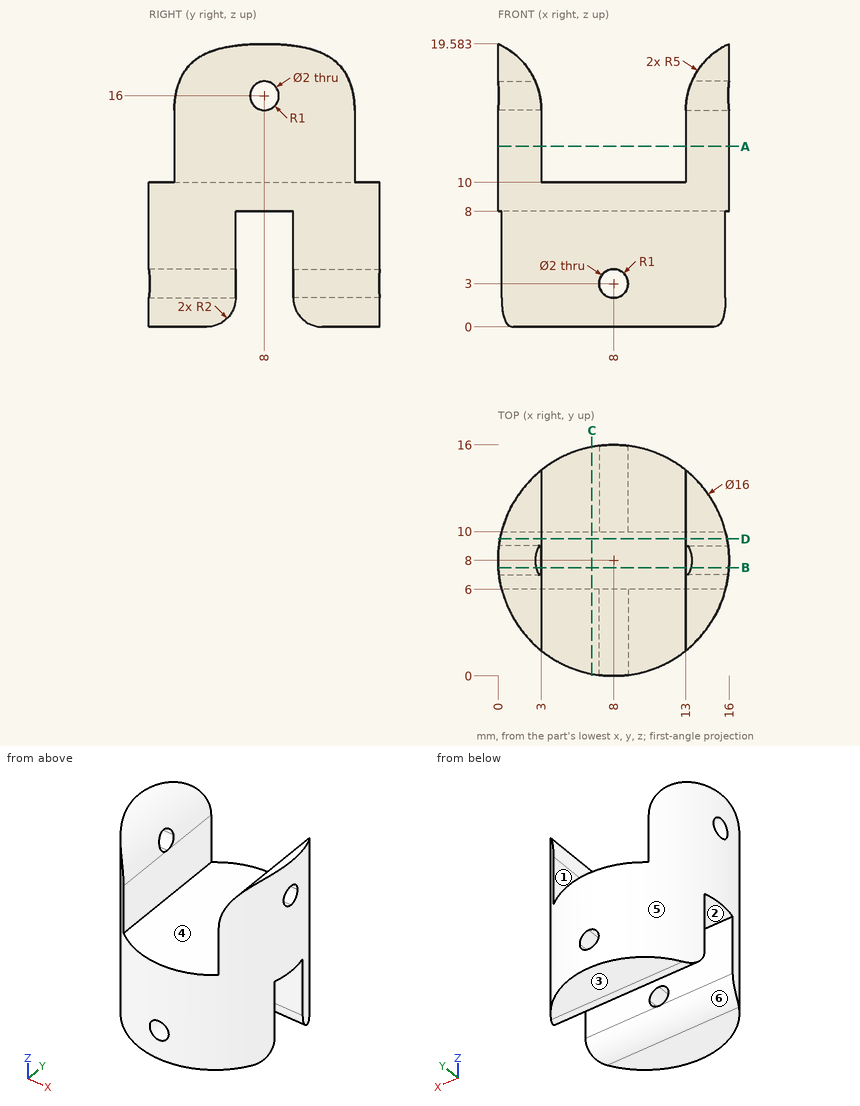
Study the drawing (mm; zero at the part's minimum x, y, z) and answer. A direction names the side the tool comes from. Coordinates: 2 decimals unless noted, no trailing zeros. Write each loop counter-clockwise with the first axis right and the second up, starting at its lowest first coordinate (ties: lowest second). Pieces come first, ordered by that corner, then holes. Notation, with made-up numbers: (23.5, 13) -> (47.5, 13) arc R4 cw to (47.5, 18) -> close; hole circle Ø4 at (3.25, 22.25). An arc over 180 degrees is marked (long way). Write item = value, one per line.
(1) Which of the six approach directions +Z, -Z, +X, -X, +Y, -Y give full straight-line access (tool end or side, diameter ignored) to the marked faces 1, 2 and 3?
From the geometry:
face_1 = +Z, +Y, -Y
face_2 = -Z, +X, -X
face_3 = -Z, +X, -X, +Y, -Y
(2) Section D-D on y = 9.5 is taken. Write down the section's boundary in (x, z).
From the geometry:
outline = (0.14, 8) -> (15.86, 8) -> (15.86, 19.52) arc R5 ccw to (13, 15) -> (13, 10) -> (3, 10) -> (3, 15) arc R5 ccw to (0.14, 19.52) -> close
(3) Section C-C on x = 6.5 is taken. Write down the section's boundary in (y, z).
From the geometry:
outline = (0.14, 0) -> (4, 0) arc R2 ccw to (6, 2) -> (6, 8) -> (10, 8) -> (10, 2) arc R2 ccw to (12, 0) -> (15.86, 0) -> (15.86, 10) -> (0.14, 10) -> close
(4) Section B-B on y = 7.5 is taken. Count the separate pieces of the cut face and the enclosed holes in it.
From the geometry:
separate_pieces = 3
enclosed_holes = 0
(5) Section A-A on z = 12.5 is taken. Write down the section's boundary in (x, y) (1 decimal).
From the geometry:
outline = (3, 1.8) -> (3, 14.2) arc R8 ccw to start; (13, 1.8) arc R8 ccw to (13, 14.2) -> close
(6) For a pull along Y with two mould halves and no side action, classify the marked faces 4, 5 and 6 as +Y half, -Y half, draft (parallel to the pull), parting line (faces both ways), or undercut.
From the geometry:
face_4 = draft
face_5 = parting line
face_6 = undercut
(7) Given pin 1 Ø6.5 at (x, z) = (11.5, 5.5) entering from -Y; pin 2 Ø8 at (x, z) = (13.5, 3.5) entering from +Y; pin 3 Ø1.8 at (y, z) = (8, 16) entering from -X; pin 4 Ø4 at (y, z) = (10.5, 12) entering from +X, each flat-ended and moving along its own axis, determine where each tip first touches the part or whether it passes through.
From the geometry:
pin_1 = 0
pin_2 = 15.86
pin_3 = through
pin_4 = 15.98
(8) Straight lines are drawn through the part: L1, parallel to Z at x = 5.5, y = 13; L2, parallel to X at y = 11, z = 2.75 (1 decimal); L3, parallel to Y at x = 7.5, z = 5.5 (1 decimal). For each, find the intervals that lie inside material, in ascending order. Write a range as from..to.
From the geometry:
L1 = 0..10
L2 = 0.6..7, 9..15.4
L3 = 0..6, 10..16
